Input: dimensioned drawing with shaded views. Units: mm. Origin: part minimum x, y, z. A direction names the side the tool comes from. Coordinates: 2 decimals unless noted, no trailing zeros. Write each loop counter-clockwise with the first axis right and the second up, starting at its lowest first coordinate (ties: lowest second). Pieces come first, ordered by that corner, then holes. Notation, with made-up numbers: (45.5, -17.5) - (57.5, -17.5) arc R18 cw to (57.5, 5.5) - close; hole circle Ø5 at (12.25, 87.5). An arc over 180 degrees is marked (long way). One line per question, with ' | ' between items.
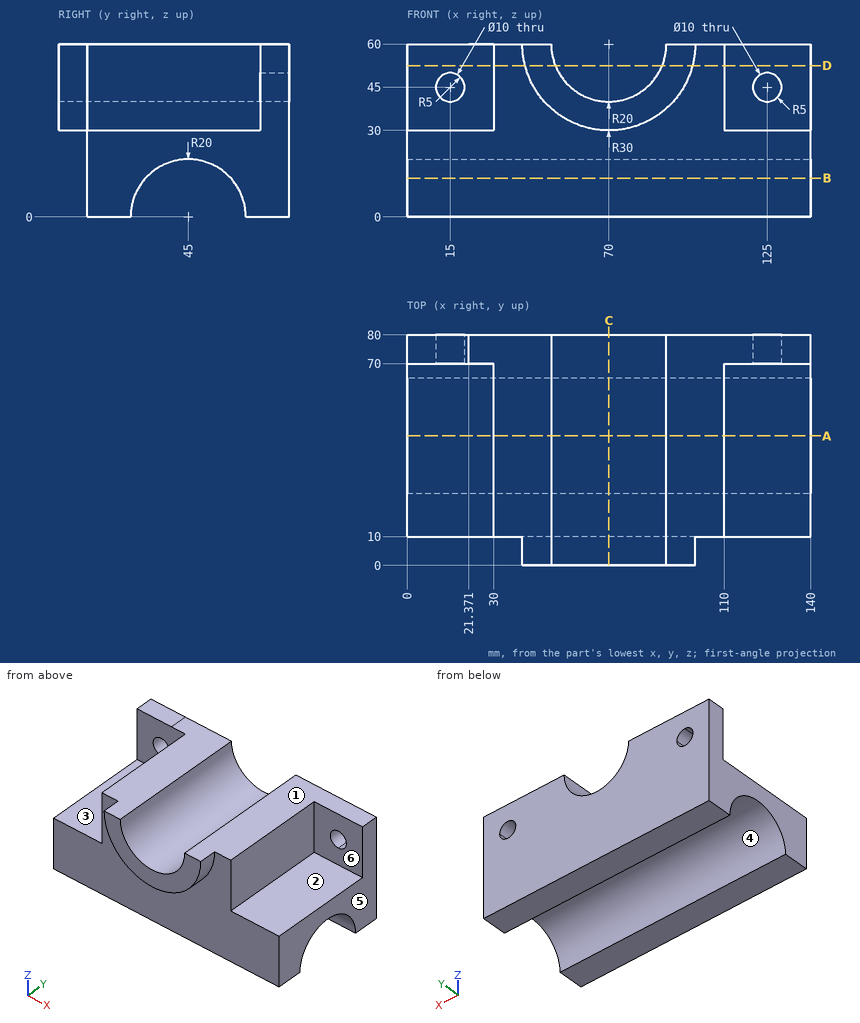
Item 1: Cut plane A-A on y = 45. Return loops of the section in (x, z).
Check sheet entries:
outline: (0, 20) - (140, 20) - (140, 30) - (110, 30) - (110, 60) - (90, 60) arc R20 cw to (50, 60) - (30, 60) - (30, 30) - (0, 30) - close
Item 2: Ray query, line 1 along X through (y, z) = (77, 45); line 2 along Z through (x, y) = (125, 75.5); line 3 along Y through (x, z) = (21.5, 40.5). Return the intervals inside material, ascending. Write a range as [from, to].
Check sheet entries:
line 1: [0, 10], [20, 56.77], [83.23, 120], [130, 140] | line 2: [0, 40], [50, 60] | line 3: [70, 80]
Item 3: Cut plane D-D on z = 52.5. Return loops of the section in (x, y).
Check sheet entries:
outline: (0, 70) - (30, 70) - (30, 10) - (40.95, 10) - (40.95, 0) - (51.46, 0) - (51.46, 80) - (0, 80) - close; (88.54, 0) - (99.05, 0) - (99.05, 10) - (110, 10) - (110, 70) - (140, 70) - (140, 80) - (88.54, 80) - close
Item 4: Mould query, pull axis Y, two halves, no side actions, for the marked faces 4, 5 and 6. Classes: pulls with the +Y half, pulls with the -Y half, needs draft (parallel to the pull), parting line crosses it, or undercut.
Check sheet entries:
face 4: undercut | face 5: needs draft | face 6: pulls with the -Y half
Item 5: Pin query (flat end, axial travel): pin 1 Ø9 at (y, z) = (28, 44.5) entering from -X; pin 2 Ø5 at (x, y) = (82, 56) entering from +Z (1 decimal); pin 3 Ø13 at (x, z) = (15, 45) entering from -Y. Return the tip coordinate at first contact, or that it passes through.
Check sheet entries:
pin 1: x = 30 | pin 2: z = 46.2 | pin 3: y = 70
Item 6: Cut plane B-B on z = 13.5. Return loops of the section in (x, y).
Check sheet entries:
outline: (0, 10) - (140, 10) - (140, 30.24) - (0, 30.24) - close; (0, 59.76) - (140, 59.76) - (140, 80) - (0, 80) - close
Item 7: Access query for the marked faces 1, 2 and 3. Directions: +Z, -Z, +X, -X, +Y, -Y. A direction counts if a zero-diameter tool reaches every point of the face in a straight line with its end or side. Return the directions, or none.
Check sheet entries:
face 1: +Z, +X, -X, +Y, -Y | face 2: +Z, +X, -Y | face 3: +Z, -X, -Y
Item 8: Cut plane C-C on x = 70. Return loops of the section in (y, z).
Check sheet entries:
outline: (0, 30) - (10, 30) - (10, 0) - (25, 0) arc R20 cw to (65, 0) - (80, 0) - (80, 40) - (0, 40) - close
